```python
from build123d import *

# Parameters (mm, degrees)
SKETCH1_R              = 64
SKETCH1_R_2            = 60
RIM_DEPTH              = 28
SKETCH2_R              = 65.5
SKETCH2_R_2            = 63
INNER_BEAD_LIP_DEPTH   = 1.5
SKETCH3_R              = 65.5
SKETCH3_R_2            = 63
OUTER_BEAD_LIP_DEPTH   = 1.5
SKETCH4_R              = 61
WEB_DEPTH              = 7
SKETCH5_R              = 8
HUB_BOSS_DEPTH         = 24
SKETCH6_R              = 13
LIGHTENING_HOLES_DEPTH = 9
SKETCH7_R              = 3.15
ROUND_BORE_6MM_DEPTH   = 30
SKETCH9_R              = 69
SKETCH9_R_2            = 64
BED_RING_DEPTH         = 1.5
SKETCH10_R             = 1.3
GRUB_SCREW_M3_DEPTH    = 9
SKETCH11_R             = 1.9
GRUB_KEY_ACCESS_DEPTH  = 62.5


with BuildPart() as part:
    # Sketch1 → Rim (new body)
    with BuildSketch(Plane.XY):
        Circle(SKETCH1_R)
        Circle(SKETCH1_R_2, mode=Mode.SUBTRACT)
    extrude(amount=RIM_DEPTH)

    # Sketch2 → Inner_bead_lip (add)
    with BuildSketch(Plane.XY):
        Circle(SKETCH2_R)
        Circle(SKETCH2_R_2, mode=Mode.SUBTRACT)
    extrude(amount=INNER_BEAD_LIP_DEPTH)

    # Sketch3 → Outer_bead_lip (add)
    with BuildSketch(Plane.XY.offset(26.5)):
        Circle(SKETCH3_R)
        Circle(SKETCH3_R_2, mode=Mode.SUBTRACT)
    extrude(amount=OUTER_BEAD_LIP_DEPTH)

    # Sketch4 → Web (add)
    with BuildSketch(Plane.XY):
        Circle(SKETCH4_R)
    extrude(amount=WEB_DEPTH)

    # Sketch5 → Hub_boss (add)
    with BuildSketch(Plane.XY):
        Circle(SKETCH5_R)
    extrude(amount=HUB_BOSS_DEPTH)

    # Sketch6 → Lightening_holes (cut)
    with BuildSketch(Plane.XY.offset(-1)):
        with Locations((32.04293994, 18.5)):
            Circle(SKETCH6_R)
        with Locations((0, 37)):
            Circle(SKETCH6_R)
        with Locations((-32.04293994, 18.5)):
            Circle(SKETCH6_R)
        with Locations((-32.04293994, -18.5)):
            Circle(SKETCH6_R)
        with Locations((0, -37)):
            Circle(SKETCH6_R)
        with Locations((32.04293994, -18.5)):
            Circle(SKETCH6_R)
    extrude(amount=LIGHTENING_HOLES_DEPTH, mode=Mode.SUBTRACT)

    # Sketch7 → Round_bore_6mm (cut)
    with BuildSketch(Plane.XY.offset(-1)):
        Circle(SKETCH7_R)
    extrude(amount=ROUND_BORE_6MM_DEPTH, mode=Mode.SUBTRACT)

    # Sketch8 → Tyre (revolve)
    with BuildSketch(Plane(origin=(0, 0, 0), x_dir=(0, 0, -1), z_dir=(1, 0, 0)), mode=Mode.PRIVATE) as tyre_sk:
        Polygon((-1.5, 64), (-26.5, 64), (-26.5, 69), (-25.5, 70), (-19, 70), (-19, 68.8), (-17, 68.8), (-17, 70), (-11, 70), (-11, 68.8), (-9, 68.8), (-9, 70), (-2.5, 70), (-1.5, 69), align=None)
    revolve(tyre_sk.sketch.rotate(Axis((0, 0, 0), (0, 0, 1)), 90), axis=Axis((0, 0, 0), (0, 0, 1)))

    # Sketch9 → Bed_ring (add)
    with BuildSketch(Plane.XY):
        with Locations(Location((0, 0, 0), (0, 0, 180))):
            Circle(SKETCH9_R)
        Circle(SKETCH9_R_2, mode=Mode.SUBTRACT)
    extrude(amount=BED_RING_DEPTH)

    # Sketch10 → Grub_screw_M3 (cut)
    with BuildSketch(Plane(origin=(0, 0, 0), x_dir=(0, 0, -1), z_dir=(1, 0, 0))):
        with Locations((-3.6, 0)):
            Circle(SKETCH10_R)
    extrude(amount=GRUB_SCREW_M3_DEPTH, mode=Mode.SUBTRACT)

    # Sketch11 → Grub_key_access (cut)
    with BuildSketch(Plane(origin=(8.5, 0, 0), x_dir=(0, 0, -1), z_dir=(1, 0, 0))):
        with Locations(Location((-3.6, 0, 0), (0, 0, 54.623459848))):
            Circle(SKETCH11_R)
    extrude(amount=GRUB_KEY_ACCESS_DEPTH, mode=Mode.SUBTRACT)


solid = part.part
```
Check sheet for the modelled part. Datum: model origin and axes. Units: mm. A direction names the side the tool comes from. Coordinates: 2 decimals unless noted, no trailing zeros. Loops run counter-clockwise (first coordinate to the right, second up) from the corner with the lowest first, then second, coordinate; pieces in that order, holes last. Notation, with made-up numbers: M 32.5,10 L 48.5,10 A28 ccw 48.5,33 Z; hole C 11,69 d4. An arc over 180 degrees is marked long. Answer as a JSON object with one key per item and string values.
1. Scan lines: L1, parallel to Y at x = 0, z = 22.25; L2, parallel to Y at x = 0, z = 3.5; L3, parallel to X at y = -18, z = 3.5. Record each from-to range of solid material in increasing order. Write a range as from..to.
Outcome:
{"L1": "-70..-60, -8..-3.15, 3.15..8, 60..70", "L2": "-70..-50, -24..-3.15, 3.15..24, 50..70", "L3": "-67.65..-45.03, -19.05..19.05, 45.03..67.65"}
2. Depth check by flat-ended pin: P1, Ø8, axis at x = 43.5, z = 16, coming from the +Y side; P2, Ø12, axis at x = -17, z = 5.5, coming from the -Y side; P3, Ø13, axis at x = -1, y = -2.5, coming from the +Z side; P4, Ø23.5, axis at x = 0, y = -37, coming from the -Z side. Enter the tip coordinate at first touch or a pass-through.
Outcome:
{"P1": "y = 57.79", "P2": "y = -69.13", "P3": "z = 24", "P4": "through"}
3. Release check for a two-part mould opening along Z. For faces 1 (the cylindrical face through (68.733, -3.025, 17.986)), 2 (the flat face through (12, 1, 7)), 3 (the cylindrical face through (15.175, 68.335, 22.204)) record: pulls with the +Z half, pulls with the -Z half, needs draft (parallel to the pull), parting line crosses it, or undercut.
Outcome:
{"face 1": "undercut", "face 2": "pulls with the +Z half", "face 3": "needs draft"}
4. Sectioned sample at B-B on x = 0. Count the separate pieces of the cut face and the enclosed holes in it, and give its area (3 significant figures).
Outcome:
{"separate pieces": "4", "enclosed holes": "0", "area": "1,130 mm²"}
5. Sectioned sample at A-A on z = 21.5. Record the cut outline in (x, y), and give its area (3 significant figures).
Outcome:
{"outline": "C 0,0 d140; C 0,0 d16; hole C 0,0 d120; hole C 0,0 d6.3", "area": "4,250 mm²"}
6. Access from +Z, -Z, +X, -X, +Y, -Y to the whole of each face (thin tool, end or side, straight path). Record for faces 4 (the flat face through (-14, -1, 0)), 5 (the flat face through (3.4, 0.1, 24)), 6 (the cylindrical face through (68.933, -3.034, 0.74)), 7 (the cylindrical face through (-3.147, 0.138, 11.832)), 8 (the flat face through (-52, 46, 19)).
Outcome:
{"face 4": "-Z, +X, -X, +Y, -Y", "face 5": "+Z", "face 6": "-Z", "face 7": "+Z, -Z", "face 8": "none"}
